from build123d import *

# Parameters (mm, degrees)
F0_R     = 12.7
F1_DEPTH = 25.4
F2_R     = 12.7
F3_DEPTH = 25.4
F4_R     = 12.7


with BuildPart() as f1:
    # F0 (on Front) → F1 (new body)
    with BuildSketch(Plane.XZ):
        with BuildLine():
            Line((56.1041173697, 12.7), (-31.2580095022, 71.8343283417))
            ThreePointArc((-31.2580095022, 71.8343283417), (-57.402141962, 73.2365993129), (-70.8958826303, 50.8))
            Line((-70.8958826303, 50.8), (-70.8958826303, 0))
            Line((-70.8958826303, 0), (56.1041173697, 0))
            Line((56.1041173697, 0), (56.1041173697, 12.7))
        make_face()
        with Locations((-45.4958826303, 50.8)):
            Circle(F0_R, mode=Mode.SUBTRACT)
    extrude(amount=F1_DEPTH)

    # F2 (on face) → F3 (join)
    with BuildSketch(Plane.XZ.offset(25.4)):
        with BuildLine():
            Line((-20.1558080966, 12.7), (-20.1558080966, 49.0562618815))
            ThreePointArc((-20.1558080966, 49.0562618815), (-22.663590516, 61.9286313985), (-31.2580095022, 71.8343283417))
            ThreePointArc((-31.2580095022, 71.8343283417), (-57.402141962, 73.2365993129), (-70.8958826303, 50.8))
            Line((-70.8958826303, 50.8), (-70.8958826303, 12.7))
            Line((-70.8958826303, 12.7), (-70.8958826303, 7.7714477666))
            Line((-70.8958826303, 7.7714477666), (-70.8958826303, 0))
            Line((-70.8958826303, 0), (56.1041173697, 0))
            Line((56.1041173697, 0), (56.1041173697, 7.7714477666))
            Line((56.1041173697, 7.7714477666), (56.1041173697, 12.7))
            Line((56.1041173697, 12.7), (-20.1558080966, 12.7))
        make_face()
        with Locations((-45.4958826303, 50.8)):
            Circle(F2_R, mode=Mode.SUBTRACT)
    extrude(amount=F3_DEPTH)

    # F4
    f4_edges = [f1.edges().sort_by_distance(p)[0] for p in [
        (56.104117, -50.8, 6.35),
    ]]
    fillet(f4_edges, radius=F4_R)


solid = f1.part
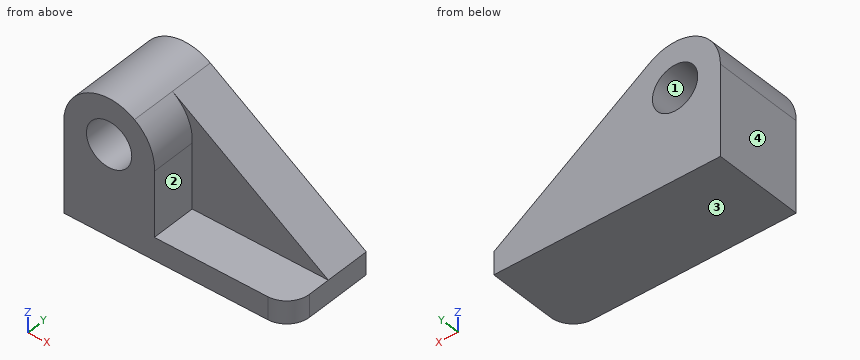
Here's how the part is built. I have some questions about the finished solid (model axes, mm). Face numbers are marked on the shaded views. Coordinates: 2 decimals unless noted, no trailing zeros. Write each loop counter-clockwise with the first axis right and the second up, starting at its lowest first coordinate (ties: lowest second). Pieces come first, ordered by that corner, then holes.
1) I'm going to push flat-ended pins straight in: pin 1 (1 mm diameter, centred on y = -36.5, z = 54.5, fed in from +X); pin 2 (1.5 mm diameter, centred on y = -24.5, z = 58, fed in from +X); pin 3 (4 mm diameter, centred on y = -5.5, z = 17, fed in from +X). Where does each tip first touch, or does it pass through?
Filled in:
pin 1: stops at x = -20.3
pin 2: stops at x = -9.71
pin 3: stops at x = 52.71
2) If we section it at D-D (y = -35.5): List the corners of the cut face in (x, z) for me, plus the area to 3 significant figures.
Filled in:
outline: (-70.9, 0) - (56.1, 0) - (56.1, 12.7) - (-20.16, 12.7) - (-20.16, 49.06) arc R25.4 ccw (long way) to (-70.9, 50.8) - close; hole circle Ø25.4 at (-45.5, 50.8)
area: 4,050 mm2
3) If we section it at C-C (z = 59.5): List the corners of the cut face in (x, y) for me.
Filled in:
outline: (-69.36, -50.8) - (-54.75, -50.8) - (-54.75, 0) - (-69.36, 0) - close; (-36.24, -50.8) - (-21.63, -50.8) - (-21.63, -25.4) - (-13.04, -25.4) - (-13.04, 0) - (-36.24, 0) - close
4) If we section it at A-A (y = -20): List the corners of the cut face in (x, z) for me, plus the area to 3 significant figures.
Filled in:
outline: (-70.9, 0) - (56.1, 0) - (56.1, 12.7) - (-31.26, 71.83) arc R25.4 ccw to (-70.9, 50.8) - close; hole circle Ø25.4 at (-45.5, 50.8)
area: 6,050 mm2
5) If I drill on line 1 (X direction, y = -28, z = 50); line 2 (Z direction, x = -15, y = -43); line 3 (X direction, y = -19.5, z = 61.5), over which ranges is the centre line in solid material (lowest first)?
Filled in:
line 1: x = -70.9 to -58.17, -32.82 to -20.11
line 2: z = 0 to 12.7
line 3: x = -68.53 to -52.34, -38.65 to -15.99
6) If we section it at B-B (x = -54.5): List the corners of the cut face in (y, z) for me.
Filled in:
outline: (-50.8, 0) - (0, 0) - (0, 41.84) - (-50.8, 41.84) - close; (-50.8, 59.76) - (0, 59.76) - (0, 74.55) - (-50.8, 74.55) - close
7) Thinking about a two-plate mould opening in X: for the marked faces 1, 2, 3 and 4, which applies, +X half, -X half, draft (parallel to the pull), parting line (faces both ways), or undercut?
Filled in:
face 1: undercut
face 2: +X half
face 3: draft
face 4: -X half
